Autodesk Inventor part; units mm, degrees
ref_plane "XZ Plane" through (0, 0, 0) normal (0, 1, 0) x (-1, 0, 0)
ref_plane "XY Plane" through (0, 0, 0) normal (0, 0, 1) x (1, 0, 0)
sketch "Sketch1" plane through (0, 0, 0) normal (0, 1, 0) x (-1, 0, 0)
  circle A0 centre (0, 0) radius 12.5
  dimension "d0" = 25
extrude "Extrusion1" add sketch "Sketch1" along normal blind 1.2
sketch "Sketch3" plane through (0, 0, 0) normal (1, 0, 0) x (0, 1, 0)
  line L0 (1.2, -12.5) -> (1.2, 12.5)
  line L1 (0, -12.5) -> (0, 12.5)
  line L2 (1.2, 10) -> (21.2, 10)
  line L3 (21.2, 10) -> (21.2, -10)
  line L4 (21.2, -10) -> (1.2, -10)
  line L5 (1.2, -10) -> (1.2, 10)
  circle A0 centre (11.2, 0) radius 7.5
  point P0 (0, 0)
  point P1 (1.2, -10)
  point P2 (1.2, -10)
  dimension "d3" = 20
  dimension "d4" = 20
  dimension "d5" = 2.5
  dimension "d6" = 15
extrude "Extrusion2" add sketch "Sketch3" along normal mid plane 4
sketch "Sketch4" plane through (2, 0, 0) normal (1, 0, 0) x (0, 0, -1)
  line L0 (-10, 21.2) -> (-10, 1.2)
  line L1 (10, 1.2) -> (-10, 1.2)
  line L2 (10, 1.2) -> (10, 21.2)
  line L3 (10, 21.2) -> (-10, 21.2)
  circle A0 centre (0, 11.2) radius 7.5
  circle A1 centre (0, 11.2) radius 7.5
  point P0 (0, 0)
extrude "Extrusion3" add sketch "Sketch4" against normal blind 0.4 contours A0
sketch "Sketch5" plane through (1.6, 11.2, 0) normal (-1, 0, 0) x (0, 0, 1)
  line L0 (10, -10) -> (10, 10)
  line L1 (10, 10) -> (-10, 10)
  line L2 (-10, 10) -> (-10, -10)
  line L3 (10, -10) -> (-10, -10)
  circle A0 centre (0, 0) radius 7.5
  circle A1 centre (0, 0) radius 2.5
  point P0 (0, -11.2)
  point P1 (0.000179, -7.5)
  dimension "d17" = 5
extrude "Extrusion4" add sketch "Sketch5" along normal up to surface (3.6 mm away) contours A1
sketch "Sketch7" plane through (-2, 11.2, 0) normal (-1, 0, 0) x (0, 0, 1)
  circle A0 centre (0, 0) radius 7.5
  line L0 (-0.006904, -7.499997) -> (2.356254, -0.835503)
  line L1 (-0.006904, -7.499997) -> (-2.357789, -0.831163)
  circle A1 centre (0, 0) radius 2.5
  circle A2 centre (0, 0) radius 2.5
  point P0 (0, -11.2)
  point P1 (2.356254, -0.835503)
  point P2 (-2.357789, -0.831163)
sketch "Sketch7 outline for Extrusion5" plane through (-2, 11.2, 0) normal (-1, 0, 0) x (0, 0, 1)
  arc A0 (2.356254, -0.835503) -> (-2.357789, -0.831163) centre (0, 0) cw
  line L0 (-0.006904, -7.499997) -> (2.356254, -0.835503)
  line L1 (-2.357789, -0.831163) -> (-0.006904, -7.499997)
extrude "Extrusion5" add sketch "Sketch7 outline for Extrusion5" against normal blind 0.8
properties part number "TestBushButton"
Read the model definition and answer for the solid it produces. Units are mm, in the model's axes. A direction names the side the tool comes from. Round coordinates to 2 decimals unless told otherwise and drop trailing zeros. Write each loop counter-clockwise with the first axis right and the second up, starting at its lowest first coordinate (ties: lowest second). Pieces come first, ordered by that corner, then holes. Notation, with made-up numbers: (-31, -32.75) -> (0, -32.75) arc R33 cw to (0, 4.25) -> close; hole circle Ø7 at (60, 1). An arc over 180 degrees is marked (long way). Answer in a Markdown table with one row per item. Add a question column.
1) Find section D-D, the plane z = 4.5. Determine the outline of the cut face in (x, y).
2) Find section C-C, the plane y = 11.2. Determine the outline of the cut face in (x, z), and give its area (3 significant figures).
3) Given P1, Ø5, axis at y = 6.5, z = -1, coming from the +X side; P2, Ø1, axis at x = -5.5, z = 5, coming from the +Y side; P3, Ø1, axis at x = -1, y = 5, coming from the +Z side; P4, Ø12.5, axis at x = -5, z = 2, coming from the +Y side, each flat-ended and moving along its own axis, determine where each tip first touches the part or whether it passes through.
4) Determine the mould class of faces 1 (the face through (-11.923, 0.592, -3.755)), 2 (the face through (0, 0, 0)), 3 (the face through (-0.17, 13.42, 1.15)) for opening direction Z: pulls with the +Z half, pulls with the -Z half, needs draft (parallel to the pull), parting line crosses it, or undercut.
5) Find section A-A, the plane x = 0. Determine the outline of the cut face in (y, z), and give its area (3 significant figures).
6) Find section B-B, the plane y = 6.75. Determine the outline of the cut face in (x, z).
7) Which of the six approach directions +Z, -Z, +X, -X, +Y, -Y give full straight-line access (tool end or side, diameter ignored) to faces 4 (the face through (-2, 10, 0)), 5 (the face through (0, 11, -10)), 6 (the face through (-1.2, 7, 0)), 7 (the face through (-1.61, 6.99, 1.16))?
8) Consider line 1 (Z direction, x = 0.85, y = 11.2); line 2 (Y direction, x = 0.15, z = 0); line 3 (X direction, y = 10.5, z = 4.25). Determine where each line is inside the solid, lowest interval first.
Findings below:
| question | item | result |
|---|---|---|
| 1 | outline | (-11.66, 0) -> (11.66, 0) -> (11.66, 1.2) -> (2, 1.2) -> (2, 21.2) -> (-2, 21.2) -> (-2, 17.2) -> (1.6, 17.2) -> (1.6, 5.2) -> (-2, 5.2) -> (-2, 1.2) -> (-11.66, 1.2) -> close |
| 2 | outline | (-2, -10) -> (2, -10) -> (2, 10) -> (-2, 10) -> (-2, 7.5) -> (1.6, 7.5) -> (1.6, 2.5) -> (-2, 2.5) -> (-2, -2.5) -> (1.6, -2.5) -> (1.6, -7.5) -> (-2, -7.5) -> close |
| 2 | area | 44.0 mm² |
| 3 | P1 | x = 2 |
| 3 | P2 | y = 1.2 |
| 3 | P3 | z = 10 |
| 3 | P4 | y = 21.2 |
| 4 | face 1 | parting line crosses it |
| 4 | face 2 | needs draft |
| 4 | face 3 | undercut |
| 5 | outline | (0, -12.5) -> (1.2, -12.5) -> (1.2, -10) -> (21.2, -10) -> (21.2, 10) -> (1.2, 10) -> (1.2, 12.5) -> (0, 12.5) -> close; circle Ø5 at (11.2, 0); hole circle Ø15 at (11.2, 0) |
| 5 | area | 273 mm² |
| 6 | outline | (-2, -10) -> (2, -10) -> (2, 10) -> (-2, 10) -> (-2, 6.04) -> (1.6, 6.04) -> (1.6, -6.04) -> (-2, -6.04) -> close; (-2, -1.08) -> (-1.2, -1.08) -> (-1.2, 1.07) -> (-2, 1.07) -> close |
| 7 | face 4 | +Z, -Z, -X, +Y |
| 7 | face 5 | -Z, +X, -X, +Y |
| 7 | face 6 | none |
| 7 | face 7 | -X |
| 8 | line 1 | -10 to -7.5, -2.5 to 2.5, 7.5 to 10 |
| 8 | line 2 | 0 to 3.7, 8.7 to 13.7, 18.7 to 21.2 |
| 8 | line 3 | 1.6 to 2 |
